Verification items for this drawing (mm, ordinates from the low corner). A direction names the side the tool comes from. Round coordinates to 2 decimals unless told otherwise and drop trailing zeros. Loops run counter-clockwise (first coordinate to the right, second up) from the corner with the lowest first, then second, coordinate; pieces in that order, holes last. Notation, with made-up numbers: (-33.75, 15.5) -> (7.25, 15.5) arc R10 cw to (7.25, 31.5) -> close; hole circle Ø2 at (1, 65.25). An arc over 180 degrees is marked (long way). One line per question, with ' | ' between items.
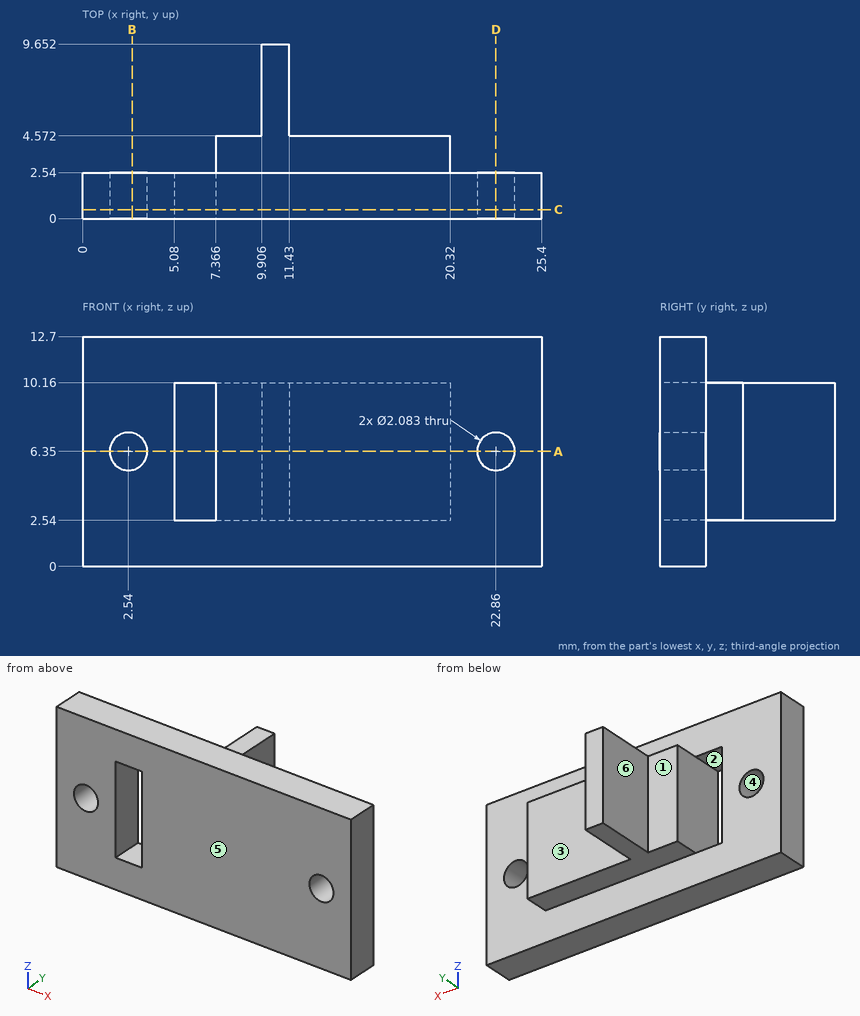
(1) Go/stop test with flat-tipped pins: pin 1 (3.5 mm diameter, centred on x = 22.86, z = 6.35, fed in from +Y); pin 2 (1.5 mm diameter, centred on y = 6, z = 7.5, fed in from +X); pin 3 (1.2 mm diameter, centred on x = 2.54, z = 6.35, fed in from -Y); pin 4 (4 mm diameter, centred on y = 6, z = 6, fed in from +X). Record where each tip stops, or that it passes through.
Answer:
pin 1: stops at y = 2.54 | pin 2: stops at x = 11.43 | pin 3: passes through | pin 4: stops at x = 20.32
(2) Sectioned sample at A-A, the plane z = 6.35. Record the cut outline in (x, y), and give its area (3 significant figures).
Answer:
outline: (0, 0) -> (1.5, 0) -> (1.5, 2.54) -> (0, 2.54) -> close; (3.58, 0) -> (5.08, 0) -> (5.08, 2.54) -> (3.58, 2.54) -> close; (7.37, 0) -> (21.82, 0) -> (21.82, 2.54) -> (20.32, 2.54) -> (20.32, 4.57) -> (11.43, 4.57) -> (11.43, 9.65) -> (9.91, 9.65) -> (9.91, 4.57) -> (7.37, 4.57) -> close; (23.9, 0) -> (25.4, 0) -> (25.4, 2.54) -> (23.9, 2.54) -> close | area: 82.2 mm2
(3) Sectioned sample at C-C, the plane y = 0.5. Record the cut outline in (x, z), and give its area (3 significant figures).
Answer:
outline: (0, 0) -> (25.4, 0) -> (25.4, 12.7) -> (0, 12.7) -> close; hole circle Ø2.08 at (2.54, 6.35); hole (5.08, 2.54) -> (7.37, 2.54) -> (7.37, 10.16) -> (5.08, 10.16) -> close; hole circle Ø2.08 at (22.86, 6.35) | area: 298 mm2
(4) Sectioned sample at D-D, the plane x = 22.86. Record the cut outline in (y, z).
Answer:
outline: (0, 0) -> (2.54, 0) -> (2.54, 5.31) -> (0, 5.31) -> close; (0, 7.39) -> (2.54, 7.39) -> (2.54, 12.7) -> (0, 12.7) -> close
(5) Set-up check for the marked faces 1, 2 and 3: record each of +Z, -Z, +X, -X, +Y, -Y from which the full face is reachable in a straight line by a thin tool's end or side.
Answer:
face 1: +Z, -Z, -X, +Y | face 2: +Y, -Y | face 3: +Z, -Z, +X, +Y
(6) Scan lines: probe 1 along Z at (x, y) = (22.86, 1.6); probe 2 along X at (y, z) = (2.25, 4.5); probe 3 along Y at (x, z) = (20.5, 5.75). Record each from-to range of solid material in increasing order.
Answer:
probe 1: z = 0 to 5.31, 7.39 to 12.7 | probe 2: x = 0 to 5.08, 7.37 to 25.4 | probe 3: y = 0 to 2.54
(7) Sectioned sample at B-B, the plane x = 2.75. Record the cut outline in (y, z), and give its area (3 significant figures).
Answer:
outline: (0, 0) -> (2.54, 0) -> (2.54, 5.33) -> (0, 5.33) -> close; (0, 7.37) -> (2.54, 7.37) -> (2.54, 12.7) -> (0, 12.7) -> close | area: 27.1 mm2
(8) Mould release check, pull along X, two halves, no side actions. Record for the marked faces 4, 5 and 6: +X half, -X half, draft (parallel to the pull), parting line (faces both ways), or undercut.
Answer:
face 4: undercut | face 5: draft | face 6: -X half
